Geometry check sheet. Reference: the model listing, model coordinates, mm. A direction names the side the tool comes from. Round coordinates to 2 decimals unless told otherwise and drop trailing zeros. Order: outer loops, then holes, each group sorted by start corner. A loop starts at its lowest first (then second) coordinate and runs counter-clockwise, first axis right, second up.
(1) Gauge pin test, flat ends, axial feed: P1, Ø2, axis at x = -5, z = -12, coming from the +Y side; P2, Ø10, axis at x = -7.5, y = 11, coming from the -Z side; P3, Ø1.5, axis at y = -11, z = -58, coming from the +X side; P4, Ø6, axis at x = 11.5, z = -58.5, coming from the -Y side. Record the tip position at first contact, or that the pin passes through.
(2) Set-up check for faces 4 (the face through (-1, 17, -30.134)), 5 (the face through (17.233, -0.758, -26.437)), 6 (the face through (8.771, -8.043, -60.487)), 7 (the face through (2.038, 9.176, -5.379)): record each of +Z, -Z, +X, -X, +Y, -Y from which the full face is reachable in a straight line by a thin tool's end or side.
(3) Cross-section at B-B on z = -25. Enter the section's corners in (x, y), and give its area (3 significant figures).
(4) Cross-section at A-A on z = -38.5. Enter the section's corners in (x, y), and give its area (3 significant figures).
(5) Draft check along Y on faces 1 (the face through (0, 0, -63.98)), 2 (the face through (-11.923, -3.755, -62.501)), 3 (the face through (-5, 0, -64.98)). Enter one of: pulls with the +Y half, pulls with the -Y half, needs draft (parallel to the pull), parting line crosses it, or undercut.
(6) Thickness scan on L1, parallel to Y at x = 0, z = -64.35; L2, parallel to Z at x = -2.5, y = 12; L3, parallel to Z at x = 6, y = 7. Record the ranges inside material, lowest first.
from build123d import *

# Parameters (mm, degrees)
SKETCH2_R          = 4.75
CUT_EXTRUDE1_DEPTH = 1


with BuildPart() as part:
    # Sketch1 → Revolve1 (revolve)
    with BuildSketch(Plane(origin=(0, 0, 0), x_dir=(1, 0, 0), z_dir=(0, 1, 0)), mode=Mode.PRIVATE) as revolve1_sk:
        Polygon((0, 0.38), (4, 0.38), (9.4, 4.911138008), (9.4, 5.834147603), (10.5, 5.834147603), (15.4, 9.945735795), (15.4, 22.634147603), (17.25, 22.634147603), (17.25, 30.134147603), (16.5, 30.134147603), (16.5, 41.134147603), (15.099029854, 57.147309648), (14.25, 59.48), (13.75, 59.48), (13.75, 59.98), (11.9, 59.98), (11.9, 60.98), (12.5, 60.98), (12.5, 63.98), (11.9, 63.98), (11.9, 64.98), (0, 64.98), align=None)
    revolve(revolve1_sk.sketch.rotate(Axis((0, 0, -64.98), (0, 0, 1)), 180), axis=Axis((0, 0, -64.98), (0, 0, 1)))

    # Sketch2 → Cut-Extrude1 (cut)
    with BuildSketch(Plane(origin=(0, 0, -64.98), x_dir=(-1, 0, 0), z_dir=(0, 0, -1))):
        Circle(SKETCH2_R)
    extrude(amount=-CUT_EXTRUDE1_DEPTH, mode=Mode.SUBTRACT)


solid = part.part
Found:
1. P1: stops at y = 14.87
1. P2: stops at z = -64.98
1. P3: stops at x = 10.75
1. P4: stops at y = -12.25
2. face 4: -Z
2. face 5: +Z, -Z
2. face 6: none
2. face 7: +Z
3. outline: circle Ø34.5 at (0, 0)
3. area: 935 mm2
4. outline: circle Ø33 at (0, 0)
4. area: 855 mm2
5. face 1: undercut
5. face 2: parting line crosses it
5. face 3: needs draft
6. L1: y = -11.9 to -4.75, 4.75 to 11.9
6. L2: z = -63.98 to -60.98, -59.98 to -7.31
6. L3: z = -64.98 to -4.76
